The model under review builds one solid part; all positions refer to its coordinate system, in mm. A direction names the side the tool comes from. Round coordinates to 2 decimals unless told otherwise and drop trailing zeros. Write each loop counter-clockwise with the first axis right and the second up, starting at its lowest first coordinate (ties: lowest second). Pieces come first, ordered by that corner, then holes. Notation, with made-up numbers: (4, 81) - (55, 81) arc R14 ccw to (55, 86) - close; hole circle Ø4 at (-18, -30.5). An arc over 180 degrees is marked (long way). Use one line per item in the form item = value.
from build123d import *

# Parameters (mm, degrees)
F0_W     = 12.7
F0_H     = 13.97
F0_R     = 1.9939
F1_DEPTH = 13.97
F2_W     = 12.7
F2_H     = 12.7
F2_R     = 1.9939
F3_DEPTH = 12.7
F4_R     = 1.9939
F5_DEPTH = 25.4


with BuildPart() as f1:
    # F0 (on Top) → F1 (new body)
    with BuildSketch(Plane.XY):
        with Locations((-41.231433, 30.867646)):
            Rectangle(F0_W, F0_H)
        with Locations((-41.231433, 30.232646)):
            Circle(F0_R, mode=Mode.SUBTRACT)
    extrude(amount=F1_DEPTH)

    # F2 (on face) → F3 (cut)
    with BuildSketch(Plane.XY.offset(13.97)):
        with Locations((-41.231433, 30.232646)):
            Rectangle(F2_W, F2_H)
        with Locations((-41.231433, 30.232646)):
            Circle(F2_R, mode=Mode.SUBTRACT)
    extrude(amount=-F3_DEPTH, mode=Mode.SUBTRACT)

    # F4 (on face) → F5 (cut)
    with BuildSketch(Plane.XZ.offset(-36.582646)):
        with Locations((-41.231433, 7.62)):
            Circle(F4_R)
    extrude(amount=-F5_DEPTH, mode=Mode.SUBTRACT)


solid = f1.part
(1) Add section D-D on x = -36.75. Write out the cut boundary in (y, z), then the cut area to 3 significant figures.
Geometry results:
outline = (23.88, 0) - (37.85, 0) - (37.85, 13.97) - (36.58, 13.97) - (36.58, 1.27) - (23.88, 1.27) - close
area = 33.9 mm2
(2) To check wall thickness, follow L1, parallel to Y at x = -37.75, z = 12.5; L2, parallel to Z at x = -42, y = 26. State the ranges of each line that lie inside material, in increasing order.
Geometry results:
L1 = 36.58 to 37.85
L2 = 0 to 1.27
(3) Add section A-A on z = 7.62. Write out the cut boundary in (x, y), then the cut area to 3 significant figures.
Geometry results:
outline = (-47.58, 36.58) - (-43.23, 36.58) - (-43.23, 37.85) - (-47.58, 37.85) - close; (-39.24, 36.58) - (-34.88, 36.58) - (-34.88, 37.85) - (-39.24, 37.85) - close
area = 11.1 mm2
(4) Add section C-C on y = 29. Write out the cut boundary in (x, z), then the cut area to 3 significant figures.
Geometry results:
outline = (-47.58, 0) - (-42.8, 0) - (-42.8, 1.27) - (-47.58, 1.27) - close; (-39.66, 0) - (-34.88, 0) - (-34.88, 1.27) - (-39.66, 1.27) - close
area = 12.1 mm2
(5) Add section B-B on x = -40.5. Write out the cut boundary in (y, z).
Geometry results:
outline = (23.88, 0) - (28.38, 0) - (28.38, 1.27) - (23.88, 1.27) - close; (32.09, 0) - (37.85, 0) - (37.85, 5.77) - (36.58, 5.77) - (36.58, 1.27) - (32.09, 1.27) - close; (36.58, 9.47) - (37.85, 9.47) - (37.85, 13.97) - (36.58, 13.97) - close
(6) Machinability: for faces 1 (the flat face through (-41, 37.853, 5)), 2 (the flat face through (-43, 32, 1.27)), which of the approach directions +Z, -Z, +X, -X, +Y, -Y give a long, thin tool a straight path to every point of the face, cutting with its end or side? Answer none if there is none.
Geometry results:
face_1 = +Z, -Z, +X, -X, +Y
face_2 = +Z, +X, -X, -Y
(7) The part is to be moulded in two halves that separate along X. For faces 3 (the flat face through (-47.581, 33, 1)), 4 (the cylindrical face through (-40.16, 31.914, 0.626)), 5 (the flat face through (-34.881, 33, 1)), 6 (the flat face through (-41, 23.883, 1)), say which applies: +X half, -X half, draft (parallel to the pull), parting line (faces both ways), or undercut.
Geometry results:
face_3 = -X half
face_4 = undercut
face_5 = +X half
face_6 = draft
(8) Insertion check: P1, Ø4, axis at x = -44.5, y = 26.5, coming from the +Z side; P2, Ø4, axis at x = -39, z = 10.5, coming from the -Y side; P3, Ø3.5, axis at x = -41.23, z = 7.62, coming from the -Y side. Each pin has a flat end and moves straight along its axis. Give the tip position at first contact, or say it passes through.
Geometry results:
P1 = 1.27
P2 = 36.58
P3 = through
